from build123d import *

# Parameters (mm, degrees)
F0_W          = 4.5
F0_H          = 11.5
F0_W_2        = 0.5
F0_W_3        = 0.9
F1_DEPTH      = 8
F1_DEPTH_BACK = 8
F4_SIZE       = 0.5
F5_R          = 1.5
F6_DEPTH      = 3.45
F5_R_2        = 0.775
F7_DEPTH      = 4.45
F5_R_3        = 1
F8_DEPTH      = 2
F9_R          = 1.5
F10_DEPTH     = 11.6
F9_R_2        = 2.5
F9_R_3        = 0.5
F11_DEPTH     = 4
F12_DEPTH     = 1


with BuildPart() as f1:
    # F0 (on Top) → F1 (new body, two sides)
    with BuildSketch(Plane.XY) as f1_sk:
        with BuildLine():
            Line((-1.4, -34.95), (-1.4, -23.45))
            Line((-1.4, -23.45), (-15.5, -23.45))
            Line((-15.5, -23.45), (-15.5, -29.95))
            Line((-15.5, -29.95), (-9.85, -29.95))
            ThreePointArc((-9.85, -29.95), (-3.9700700534, -30.95), (-9.85, -31.95))
            Line((-9.85, -31.95), (-15.5, -31.95))
            Line((-15.5, -31.95), (-15.5, -34.95))
            Line((-15.5, -34.95), (-2.5, -34.95))
            Line((-2.5, -34.95), (-1.4, -34.95))
        make_face()
        with Locations((2.25, -29.2)):
            Rectangle(F0_W, F0_H)
        with Locations((-1.15, -29.2)):
            Rectangle(F0_W_2, F0_H)
        with Locations((-0.45, -29.2)):
            Rectangle(F0_W_3, F0_H)
    extrude(amount=F1_DEPTH)
    extrude(f1_sk.sketch, amount=-F1_DEPTH_BACK)

    # F0 (on Top) → F2 (revolve)
    with BuildSketch(Plane.XY):
        with Locations((-1.15, -29.2)):
            Rectangle(F0_W_2, F0_H)
        Polygon((-0.9, -38.95), (-0.9, -34.95), (-1.4, -34.95), (-2.5, -34.95), (-2.5, -35.95), (-1.9, -38.9505927906), (-0.5, -40.95), (-0.2, -40.95), align=None)
        Polygon((-0.9, -23.45), (-0.9, 14.85), (-4, 14.85), (-4, 21.35), (-8, 21.35), (-8, 17.65), (-6, 17.65), (-6, 11.65), (-8, 11.65), (-8, 8.65), (-4.5, 8.65), (-4.5, 7.15), (-8, 7.15), (-8, 6.15), (-4.5, 6.15), (-4.5, 4.65), (-11.15, 4.65), (-11.15, 3.65), (-4.75, 3.65), (-4.75, 2.15), (-11.15, 2.15), (-11.15, 1.15), (-5, 1.15), (-5, -0.35), (-11.15, -0.35), (-11.15, -1.35), (-5.25, -1.35), (-5.25, -2.85), (-11.15, -2.85), (-11.15, -3.85), (-5.5, -3.85), (-5.5, -5.35), (-11.15, -5.35), (-11.15, -6.35), (-5.75, -6.35), (-5.75, -7.85), (-11.15, -7.85), (-11.15, -8.85), (-6, -8.85), (-6, -10.35), (-11.15, -10.35), (-11.15, -11.35), (-6.25, -11.35), (-6.25, -12.85), (-11.15, -12.85), (-11.15, -13.85), (-6.5, -13.85), (-6.5, -15.35), (-11.15, -15.35), (-11.15, -16.35), (-6.75, -16.35), (-6.75, -17.85), (-11.15, -17.85), (-11.15, -18.85), (-7, -18.85), (-7, -20.35), (-11.15, -20.35), (-11.15, -21.35), (-1.4, -21.35), (-1.4, -23.45), align=None)
    revolve(axis=Axis((0, 15, 0), (0, 1, 0)))

    # F0 (on Top) → F3 (revolve, cut)
    with BuildSketch(Plane.XY):
        with Locations((-0.45, -29.2)):
            Rectangle(F0_W_3, F0_H)
    revolve(axis=Axis((0, 15, 0), (0, 1, 0)), mode=Mode.SUBTRACT)

    # F4
    f4_edges = [f1.edges().sort_by_distance(p)[0] for p in [
        (-15.5, -23.45, 0),
        (-15.5, -26.7, 8),
        (-5.5, -23.45, 8),
        (-15.5, -26.7, -8),
        (-15.5, -33.45, -8),
        (-15.5, -33.45, 8),
        (4.5, -29.2, -8),
        (-5.5, -23.45, -8),
        (-5.5, -34.95, -8),
        (-15.5, -34.95, 0),
        (4.5, -23.45, 0),
        (4.5, -34.95, 0),
        (4.5, -29.2, 8),
        (-5.5, -34.95, 8),
    ]]
    chamfer(f4_edges, length=F4_SIZE)

    # F5 (on face) → F6 (cut)
    with BuildSketch(Plane.XY.offset(8)):
        with Locations((1, -30.15)):
            Circle(F5_R)
    extrude(amount=-F6_DEPTH, mode=Mode.SUBTRACT)

    # F5 (on face) → F7 (cut)
    with BuildSketch(Plane.XY.offset(8)):
        with Locations((2.5, -32.95)):
            Circle(F5_R_2)
    extrude(amount=-F7_DEPTH, mode=Mode.SUBTRACT)

    # F5 (on face) → F8 (cut)
    with BuildSketch(Plane.XY.offset(8)):
        with Locations((2.5, -32.95)):
            Circle(F5_R_3)
        with Locations((2.5, -32.95)):
            Circle(F5_R_2, mode=Mode.SUBTRACT)
    extrude(amount=-F8_DEPTH, mode=Mode.SUBTRACT)

    # F9 (on face) → F10 (cut)
    with BuildSketch(Plane.XZ.offset(34.95)):
        with Locations((-13, 0)):
            Circle(F9_R)
    extrude(amount=-F10_DEPTH, mode=Mode.SUBTRACT)

    # F9 (on face) → F11 (join)
    with BuildSketch(Plane.XZ.offset(34.95)):
        Polygon((3.5, -2.0207259422), (3.5, 2.0207259422), (0, 4.0414518843), (-3.5, 2.0207259422), (-3.5, -2.0207259422), (0, -4.0414518843), align=None)
        Circle(F9_R_2, mode=Mode.SUBTRACT)
        Circle(F9_R_2)
        Circle(F9_R_3, mode=Mode.SUBTRACT)
    extrude(amount=F11_DEPTH)

    # F9 (on face) → F12 (cut)
    with BuildSketch(Plane.XZ.offset(34.95)):
        Polygon((3.5, -2.0207259422), (3.5, 2.0207259422), (0, 4.0414518843), (-3.5, 2.0207259422), (-3.5, -2.0207259422), (0, -4.0414518843), align=None)
        Circle(F9_R_2, mode=Mode.SUBTRACT)
    extrude(amount=F12_DEPTH, mode=Mode.SUBTRACT)


solid = f1.part
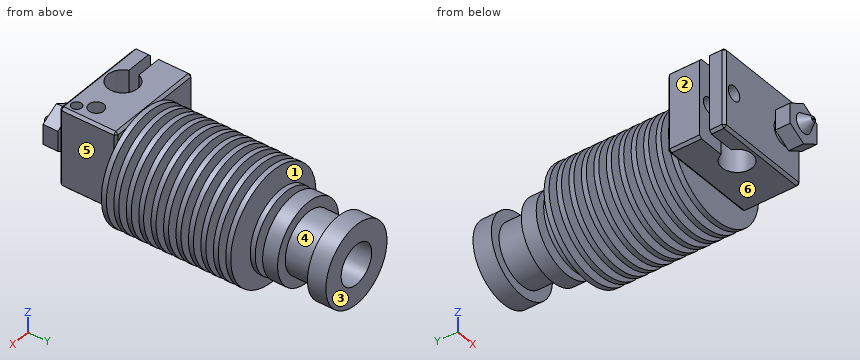
Source: CAD feature listing. Evaluate the final solid. Frame: model axes, mm. Face numbers are marked on the shaded views. A direction names the side the tool comes from. Coordinates: 2 decimals unless noted, no trailing zeros. Loops run counter-clockwise (first coordinate to the right, second up) from the corner with the lowest first, then second, coordinate; pieces in that order, holes last. Notation, with made-up numbers: M 0.5,74 L 9.5,74 A13 ccw 9.5,87 Z; hole C -25,70 d2. An arc over 180 degrees is marked long. Answer in a Markdown table with one row per item.
Q1. Section B-B on y = 15.5. Return the cut outline in (x, z), plus the area to 3 significant figures.
Answers below:
| item | result |
|---|---|
| outline | C 0,0 d12; hole C 0,0 d8 |
| area | 62.8 mm^2 |
Q2. Draft query along Y for the marked faces 1, 2 and 3. Return one class per face: pulls with the +Y half, pulls with the -Y half, needs draft (parallel to the pull), parting line crosses it, or undercut.
Answers below:
| item | result |
|---|---|
| face 1 | undercut |
| face 2 | needs draft |
| face 3 | pulls with the +Y half |
Q3. Section C-C on x = 9. State how many separate pieces and enclosed holes the cut face has, plus the area to 3 significant figures.
Answers below:
| item | result |
|---|---|
| separate pieces | 11 |
| enclosed holes | 0 |
| area | 145 mm^2 |
Q4. Set-up query: the marked faces 4, 5 and 6. Return all of +Z, -Z, +X, -X, +Y, -Y with unobstructed straight access to the full face (end or side cutting, diameter ignored); none if empty.
Answers below:
| item | result |
|---|---|
| face 4 | none |
| face 5 | +Z, -Z, +X, -Y |
| face 6 | -Z, +X, -X, -Y |
Q5. Ray query, probe 1 along Y at (x, z) = (-3.25, -3.25); probe 2 along Y at (x, z) = (2.5, 4.3) (3 decimals); probe 3 along Z at (x, y) = (-13, -34.15). Return the intervals inside material, ascending. Write a range as from..to.
Answers below:
| item | result |
|---|---|
| probe 1 | y = -34.95..-23.45, -21.35..4.65, 6.15..7.15, 8.65..21.35 |
| probe 2 | y = -34.95..-33.725, -32.175..-23.45, -21.35..2.15, 3.65..4.65, 6.15..7.15, 8.65..21.35 |
| probe 3 | z = -8..-1.5, 1.5..8 |
Q6. Section A-A on y = -32.95. Return the cut outline in (x, z) (3 decimals).
Answers below:
| item | result |
|---|---|
| outline | M -15.5,-7.5 L -15,-8 L -9.265,-8 L -9.265,8 L -15,8 L -15.5,7.5 Z; M -4.726,-8 L 4,-8 L 4.5,-7.5 L 4.5,7.5 L 4,8 L 3.5,8 L 3.5,6 L 3.275,6 L 3.275,3.55 L 1.725,3.55 L 1.725,6 L 1.5,6 L 1.5,8 L -4.726,8 Z; hole C -13,0 d3; hole C 0,0 d1.8 |
Q7. First-contact query: pin 1 (10 mm diameter, centred on x = -1, z = -7, fed in from -Y); pin 2 (8.5 mm diameter, centred on x = -2.5, y = -27.5, fed in from -Z); pin 3 (1.6 mm diameter, centred on x = 2.5, y = -33, fed in from +Z). Flat tips, straight axial feed; report the tip coordinate or a pass-through.
Answers below:
| item | result |
|---|---|
| pin 1 | stops at y = -38.95 |
| pin 2 | stops at z = -8 |
| pin 3 | stops at z = 6 |
